```python
from build123d import *

# Parameters (mm, degrees)
EXTRUDE_1_DEPTH     = 3
SKETCH_2_R          = 1.55
CUT_EXTRUDE_1_DEPTH = 10
SKETCH_3_R          = 1.55
CUT_EXTRUDE_2_DEPTH = 10


with BuildPart() as part:
    # 草图1 → 凸台-拉伸1 (new body)
    with BuildSketch(Plane(origin=(0, 0, 0), x_dir=(1, 0, 0), z_dir=(0, 1, 0))):
        Polygon((50, 45), (-50, 45), (-50, 5), (25, 5), (25, -45), (50, -45), align=None)
    extrude(amount=EXTRUDE_1_DEPTH)

    # 草图2 → 切除-拉伸1 (cut)
    with BuildSketch(Plane(origin=(0, 0, 0), x_dir=(-1, 0, 0), z_dir=(0, -1, 0))):
        with Locations(Location((5, 38, 0), (0, 0, 90))):
            Circle(SKETCH_2_R)
        with Locations(Location((5, 14, 0), (0, 0, 90))):
            Circle(SKETCH_2_R)
        with Locations(Location((35, 38, 0), (0, 0, 90))):
            Circle(SKETCH_2_R)
        with Locations(Location((35, 14, 0), (0, 0, 90))):
            Circle(SKETCH_2_R)
    extrude(amount=-CUT_EXTRUDE_1_DEPTH, mode=Mode.SUBTRACT)

    # 草图3 → 切除-拉伸2 (cut)
    with BuildSketch(Plane(origin=(0, 0, 0), x_dir=(-1, 0, 0), z_dir=(0, -1, 0))):
        with Locations(Location((-37.5, 13, 0), (0, 0, 90))):
            Circle(SKETCH_3_R)
        with Locations(Location((-37.5, -35, 0), (0, 0, 90))):
            Circle(SKETCH_3_R)
    extrude(amount=-CUT_EXTRUDE_2_DEPTH, mode=Mode.SUBTRACT)


solid = part.part
```
Verification items for the finished model (mm, model axes). A direction names the side the tool comes from. Coordinates: 2 decimals unless noted, no trailing zeros. Loops run counter-clockwise (first coordinate to the right, second up) from the corner with the lowest first, then second, coordinate; pieces in that order, holes last. Notation, with made-up numbers: (-28.75, 41) -> (25.25, 41) arc R17 ccw to (25.25, 65) -> close; hole circle Ø1 at (8, 54.5). An arc over 180 degrees is marked (long way). Answer in a Markdown table with one row per item. Add a question column.
1. Depth check by flat-ended pin: P1, Ø2.5, axis at x = -35, z = -38, coming from the -Y side; P2, Ø1.5, axis at x = 17.5, y = 2.5, coming from the +Z side. Enter the tip coordinate at first touch or a pass-through.
2. Section check A-A, the plane x = 37.5. Enter the section's corners in (y, z), then the cut area to 3 significant figures.
3. Section check D-D, the plane z = -38. Enter the section's corners in (x, y), then the cut area to 3 significant figures.
4. Draft check along X on faces 3 (the face through (-34.534, 1.479, -39.478)), 4 (the face through (-4.534, 1.479, -39.478)), 5 (the face through (50, 1, 1)), 6 (the face through (37, 1, 45)). Enter one of: +X half, -X half, draft (parallel to the pull), parting line (faces both ways), or undercut.
5. Access from +Z, -Z, +X, -X, +Y, -Y to the whole of each face (thin tool, end or side, straight path). Record for faces 1 (the face through (10, 0, -21)), 2 (the face through (25, 1, 20)).
6. Section check B-B, the plane z = 35. Enter the section's corners in (x, y), then the cut area to 3 significant figures.
7. Material ranges on probe 1 along X at (y, z) = (2.05, -38); probe 2 along X at (y, z) = (2.05, -13); probe 3 along X at (y, z) = (1.55, -14), recorded low to high. Write a range as [from, to].
8. Section check C-C, the plane y = 0.8. Enter the section's corners in (x, z), then the cut area to 3 significant figures.
Derived:
| question | item | result |
|---|---|---|
| 1 | P1 | passes through |
| 1 | P2 | stops at z = -5 |
| 2 | outline | (0, -45) -> (3, -45) -> (3, -14.55) -> (0, -14.55) -> close; (0, -11.45) -> (3, -11.45) -> (3, 33.45) -> (0, 33.45) -> close; (0, 36.55) -> (3, 36.55) -> (3, 45) -> (0, 45) -> close |
| 2 | area | 251 mm² |
| 3 | outline | (-50, 0) -> (-36.55, 0) -> (-36.55, 3) -> (-50, 3) -> close; (-33.45, 0) -> (-6.55, 0) -> (-6.55, 3) -> (-33.45, 3) -> close; (-3.45, 0) -> (50, 0) -> (50, 3) -> (-3.45, 3) -> close |
| 3 | area | 281 mm² |
| 4 | face 3 | undercut |
| 4 | face 4 | undercut |
| 4 | face 5 | +X half |
| 4 | face 6 | draft |
| 5 | face 1 | +Z, -Z, +X, -X, -Y |
| 5 | face 2 | +Z, -X, +Y, -Y |
| 6 | outline | (25, 0) -> (35.95, 0) -> (35.95, 3) -> (25, 3) -> close; (39.05, 0) -> (50, 0) -> (50, 3) -> (39.05, 3) -> close |
| 6 | area | 65.7 mm² |
| 7 | probe 1 | x = [-50, -36.55], [-33.45, -6.55], [-3.45, 50] |
| 7 | probe 2 | x = [-50, -36.18], [-33.82, -6.18], [-3.82, 35.95], [39.05, 50] |
| 7 | probe 3 | x = [-50, -36.55], [-33.45, -6.55], [-3.45, 36.32], [38.68, 50] |
| 8 | outline | (-50, -45) -> (50, -45) -> (50, 45) -> (25, 45) -> (25, -5) -> (-50, -5) -> close; hole circle Ø3.1 at (-35, -38); hole circle Ø3.1 at (-35, -14); hole circle Ø3.1 at (-5, -38); hole circle Ø3.1 at (-5, -14); hole circle Ø3.1 at (37.5, -13); hole circle Ø3.1 at (37.5, 35) |
| 8 | area | 5,200 mm² |
